Solid Edge part; units mm, degrees
sketch "Sketch1" plane through (0, 0, 0) normal (0, 0, 1) x (1, 0, 0)
  circle A0 centre (0, 0) radius 1.6
  circle A1 centre (0, 0) radius 3.5
extrude "Protrusion1" add sketch "Sketch1" along normal blind 0.5
fillet "Round_Edges" radius 0.05 4 edges at (-3.5, 0, 0.5) (-3.5, 0, 0) (-1.6, 0, 0.5) (-1.6, 0, 0)
properties material "Nylon, general purpose"
Geometry: final body of the model. Coordinates: model frame, mm. Give positions to 0.01 mm unless a question says otherwise; leave off trailing zeros. Loops run counter-clockwise (first coordinate to the right, second up) from the corner with the lowest first, then second, coordinate; pieces in that order, holes last. Notation, with made-up numbers: M -1,-31 L 16,-31 A12 cw 16,-9 Z; hole C 36.5,-27.75 d9. An arc over 180 degrees is marked long. Put each result on its own line as item: value. Start each with the question number.
1) Cut plane C-C (z = 0.25). Output: boundary loops of the cut face in (x, y).
2) Cut plane A-A (x = 0). Output: boundary loops of the cut face in (y, z), then the cut area to 3 significant figures.
3) Ray query, line 1 along Y through (x, z) = (0, 0.25); line 2 along Y through (x, z) = (-0.5, 0.1). Return the intervals inside material, ascending.
4) Pull-direction query (Y, two-part tool) for faces 1 (the cylindrical face through (3.233, 1.341, 0.247)), 2 (the cylindrical face through (-1.27, 0.97, 0.25)), 3 (the flat face through (1, 2, 0.5)); classes: pulls with the +Y half, pulls with the -Y half, needs draft (parallel to the pull), parting line crosses it, or undercut.
Verdict:
1. outline: C 0,0 d7; hole C 0,0 d3.2
2. outline: M -3.5,0.05 A0.05 ccw -3.45,0 L -1.65,0 A0.05 ccw -1.6,0.05 L -1.6,0.45 A0.05 ccw -1.65,0.5 L -3.45,0.5 A0.05 ccw -3.5,0.45 Z; M 1.6,0.05 A0.05 ccw 1.65,0 L 3.45,0 A0.05 ccw 3.5,0.05 L 3.5,0.45 A0.05 ccw 3.45,0.5 L 1.65,0.5 A0.05 ccw 1.6,0.45 Z
2. area: 1.90 mm2
3. line 1: -3.5 to -1.6, 1.6 to 3.5
3. line 2: -3.46 to -1.52, 1.52 to 3.46
4. face 1: parting line crosses it
4. face 2: undercut
4. face 3: needs draft
